Autodesk Inventor part; units mm, degrees
ref_plane "YZ Plane" through (0, 0, 0) normal (1, 0, 0) x (0, 1, 0)
ref_plane "XZ Plane" through (0, 0, 0) normal (0, 1, 0) x (-1, 0, 0)
ref_plane "XY Plane" through (0, 0, 0) normal (0, 0, 1) x (1, 0, 0)
sketch "Sketch1" plane through (0, 0, 0) normal (0, 0, 1) x (1, 0, 0)
  line L0 (0, 147) -> (0, -147)
  line L1 (-161, 0) -> (161, 0)
  line L2 (115, -105) -> (-115, -105)
  line L3 (-115, -105) -> (-115, 105)
  line L4 (-115, 105) -> (115, 105)
  line L5 (115, 105) -> (115, -105)
  line L6 (115, -105) -> (-115, 105) construction
  line L7 (-115, -105) -> (115, 105) construction
  line L8 (75, -75) -> (-75, -75) construction
  line L9 (-75, -75) -> (-75, 75) construction
  line L10 (-75, 75) -> (75, 75) construction
  line L11 (75, 75) -> (75, -75) construction
  line L12 (75, -75) -> (-75, 75) construction
  line L13 (-75, -75) -> (75, 75) construction
  line L14 (25, -25) -> (-25, -25) construction
  line L15 (-25, -25) -> (-25, 25) construction
  line L16 (-25, 25) -> (25, 25) construction
  line L17 (25, 25) -> (25, -25) construction
  line L18 (25, -25) -> (-25, 25) construction
  line L19 (-25, -25) -> (25, 25) construction
  point P0 (0, 0)
  dimension "d0" = 230
  dimension "d1" = 210
  dimension "d2" = 150
  dimension "d3" = 150
  dimension "d4" = 50
  dimension "d5" = 50
extrude "Extrusion1" add sketch "Sketch1" against normal blind 15.875
hole "Hole1" at (-75, 75, 0) at (75, 75, 0) at (75, -75, 0) at (-75, -75, 0) at (-25, 25, 0) at (25, 25, 0) at (25, -25, 0) at (-25, -25, 0) direction (0, 0, -1) diameter 7.0104 end through all counterbore diameter 12.7 counterbore depth 5.9944
sketch "Sketch2" plane through (0, 0, -15.875) normal (0, 0, -1) x (-1, 0, 0)
  line L0 (0, -147) -> (0, 147)
  line L1 (-161, 0) -> (161, 0)
  line L2 (100, -100) -> (-100, -100) construction
  line L3 (-100, -100) -> (-100, 100) construction
  line L4 (-100, 100) -> (100, 100) construction
  line L5 (100, 100) -> (100, -100) construction
  line L6 (100, -100) -> (-100, 100) construction
  line L7 (-100, -100) -> (100, 100) construction
  circle A0 centre (101.5, -27) radius 1.5 construction
  circle A1 centre (88.57, 101.5) radius 1.5 construction
  circle A2 centre (-88.57, 101.5) radius 1.5 construction
  point P0 (0, 0)
  dimension "d15" = 200
  dimension "d16" = 200
  dimension "d17" = 3
  dimension "d18" = 127
  dimension "d19" = 11.43
  dimension "d20" = 11.43
hole "Hole2" at (-101.5, -27, -15.875) at (-88.57, 101.5, -15.875) at (88.57, 101.5, -15.875) direction (0, 0, 1) diameter 2.9972 end through all counterbore diameter 3.0226 counterbore depth 1.905
chamfer "Chamfer1" distance 19.05 angle 45 2 edges at (-115, -105, -7.9375) (115, -105, -7.9375)
sketch "Sketch3" plane through (-115, 105, 0) normal (0, 1, 0) x (1, 0, 0)
  line L0 (115, 19.05) -> (115, -3.175)
  line L1 (276, 0) -> (-46, 0)
  line L2 (19.75, 7.9375) -> (210.25, 7.9375) construction
  line L3 (0, 15.875) -> (230, 15.875)
  point P0 (115, 0)
  point P1 (45.15, 7.9375)
  point P2 (184.85, 7.9375)
  dimension "d31" = 95.25
  dimension "d32" = 95.25
  dimension "d33" = 69.85
  dimension "d34" = 69.85
  dimension "d49" = 7.9375
  dimension "d50" = 15.875
hole "Hole3" at (95.25, 105, -7.9375) at (-95.25, 105, -7.9375) direction (0, -1, 0) diameter 4.9276 depth 12.7 tip angle 118
hole "Hole4" at (69.85, 105, -7.9375) at (-69.85, 105, -7.9375) direction (0, -1, 0) diameter 6.35 depth 12.7 tip angle 118 counterbore diameter 6.3754 counterbore depth 3.175
sketch "Sketch4" plane through (0, 0, 0) normal (0, 0, 1) x (1, 0, 0)
  line L0 (0, 147) -> (0, -147)
  line L1 (-161, 0) -> (161, 0)
  line L2 (-115, -85.95) -> (-115, 105)
  line L3 (115, 105) -> (115, -85.95)
  line L4 (109, 45) -> (-109, 45) construction
  line L5 (-109, 45) -> (-109, 85) construction
  line L6 (-109, 85) -> (109, 85) construction
  line L7 (109, 85) -> (109, 45) construction
  line L8 (109, 45) -> (-109, 85) construction
  line L9 (-109, 45) -> (109, 85) construction
  line L10 (-115, 105) -> (115, 105) construction
  point P0 (0, 0)
  point P1 (0, 65)
  dimension "d51" = 6
  dimension "d52" = 20
  dimension "d53" = 40
hole "Hole5" at (-109, 85, 0) at (-109, 45, 0) at (109, 45, 0) at (109, 85, 0) direction (0, 0, -1) diameter 6.604 end through all
equation "\"d49\" = 0.5 * d50"
properties part number "J008085" material "ALUMINUM, 6061-T651"
CAD build for the part. Positions are in the model's coordinates, mm. A direction names the side the tool comes from. Coordinates: 2 decimals unless noted, no trailing zeros. Order: outer loops, then holes, each group sorted by start corner. A loop starts at its lowest first (then second) coordinate and runs counter-clockwise, first axis right, second up.
(1) Saw through at C-C, the plane x = 109. Write the cut outline in (y, z) (3 decimals), and give its area (3 significant figures).
Solution:
outline: (-91.95, -15.875) - (41.698, -15.875) - (41.698, 0) - (-91.95, 0) - close; (48.302, -15.875) - (81.698, -15.875) - (81.698, 0) - (48.302, 0) - close; (88.302, -15.875) - (105, -15.875) - (105, 0) - (88.302, 0) - close
area: 2,920 mm2
(2) Saw through at B-B, the plane y = 45. Write the cut outline in (x, z) (3 decimals), and give its area (3 significant figures).
Solution:
outline: (-115, -15.875) - (-112.302, -15.875) - (-112.302, 0) - (-115, 0) - close; (-105.698, -15.875) - (105.698, -15.875) - (105.698, 0) - (-105.698, 0) - close; (112.302, -15.875) - (115, -15.875) - (115, 0) - (112.302, 0) - close
area: 3,440 mm2
(3) Saw through at A-A, the plane x = 25. Write the cut outline in (y, z) (3 decimals).
Solution:
outline: (-105, -15.875) - (-28.505, -15.875) - (-28.505, -5.994) - (-31.35, -5.994) - (-31.35, 0) - (-105, 0) - close; (-21.495, -15.875) - (21.495, -15.875) - (21.495, -5.994) - (18.65, -5.994) - (18.65, 0) - (-18.65, 0) - (-18.65, -5.994) - (-21.495, -5.994) - close; (28.505, -15.875) - (105, -15.875) - (105, 0) - (31.35, 0) - (31.35, -5.994) - (28.505, -5.994) - close
(4) Which spindle directions (+Z, -Z, +X, -X, +Y, -Y) get a long thin tool onto all of the face, cutting with end or side? Do faces 4 (the face through (-66.75, 97, -8.63)), 5 (the face through (-26.907, 18.943, -3.039)), 6 (the face through (74.8, -71.5, -11)). Say none if no direction does.
Solution:
face 4: +Y
face 5: +Z
face 6: +Z, -Z
(5) Pin check, flat tips, straight feed: pin 1 Ø10 at (x, y) = (-75, -74) entering from +Z; pin 2 Ø1.9 at (x, z) = (70.5, -6.5) entering from +Y. Stop position of each tip, or through.
Solution:
pin 1: stops at z = -5.99
pin 2: stops at y = 91.91
(6) Drill centre lines: L1, parallel to X at y = -75, z = -8.5; L2, parallel to Y at x = -25, z = -1.65; L3, parallel to Y at x = -25, z = -9.75. Where is each one in solid material? Low to high.
Solution:
L1: x = -115 to -78.51, -71.49 to 71.49, 78.51 to 115
L2: y = -105 to -31.35, -18.65 to 18.65, 31.35 to 105
L3: y = -105 to -28.51, -21.49 to 21.49, 28.51 to 105
(7) Mould opens along Z. For faces 1 (the face through (94.87, 91.077, -7.74)), 2 (the face through (78, -78, -5.994)), 3 (the face through (80.634, 72.07, -3.039)) say: released by +Z, released by -Z, zero draft, split by the parting line, or undercut.
Solution:
face 1: undercut
face 2: released by +Z
face 3: zero draft
(8) Saw through at D-D, the plane y = -75. Write the cut outline in (x, z) (3 decimals).
Solution:
outline: (-115, -15.875) - (-78.505, -15.875) - (-78.505, -5.994) - (-81.35, -5.994) - (-81.35, 0) - (-115, 0) - close; (-71.495, -15.875) - (71.495, -15.875) - (71.495, -5.994) - (68.65, -5.994) - (68.65, 0) - (-68.65, 0) - (-68.65, -5.994) - (-71.495, -5.994) - close; (78.505, -15.875) - (115, -15.875) - (115, 0) - (81.35, 0) - (81.35, -5.994) - (78.505, -5.994) - close
